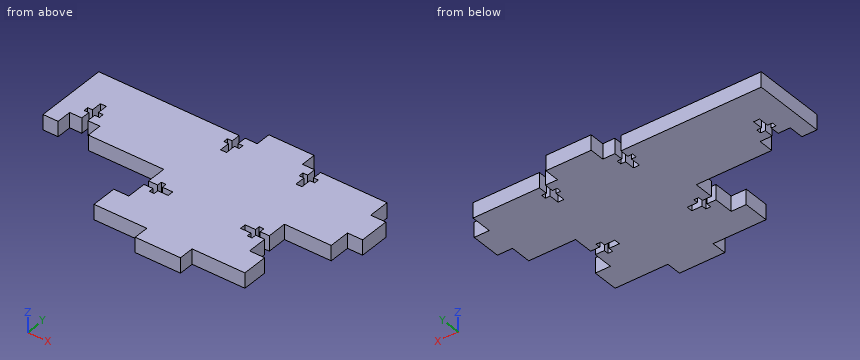
from build123d import *

# Parameters (mm, degrees)
BOSS_EXTRUDE1_DEPTH = 6.35
SKETCH2_W           = 12.7
SKETCH2_H           = 6.35
CUT_EXTRUDE1_DEPTH  = 7.35
CUT_EXTRUDE2_DEPTH  = 7.35
CUT_EXTRUDE3_DEPTH  = 7.35


with BuildPart() as part:
    # Sketch1 → Boss-Extrude1 (new body)
    with BuildSketch(Plane.XY):
        Polygon((0, -6.35), (19.05, -6.35), (19.05, 0), (34.925, 0), (41.275, 0), (41.275, 10.795), (34.925, 10.795), (34.925, 29.845), (54.61, 29.845), (54.61, 38.735), (60.96, 38.735), (60.96, 51.435), (54.61, 51.435), (54.61, 60.325), (34.925, 60.325), (19.05, 60.325), (19.05, 66.675), (0, 66.675), (0, 60.325), (-15.875, 60.325), (-66.675, 60.325), (-66.675, 29.845), (-15.875, 29.845), (-15.875, 10.795), (-22.225, 10.795), (-22.225, 0), (-15.875, 0), (0, 0), align=None)
    extrude(amount=BOSS_EXTRUDE1_DEPTH)

    # Sketch2 → Cut-Extrude1 (cut, through all)
    with BuildSketch(Plane.XY.offset(6.35)):
        with Locations((-53.975, 33.02)):
            Rectangle(SKETCH2_W, SKETCH2_H)
    extrude(amount=-CUT_EXTRUDE1_DEPTH, mode=Mode.SUBTRACT)

    # Sketch3 → Cut-Extrude2 (cut, through all)
    with BuildSketch(Plane.XY.offset(6.35)):
        Polygon((-15.875, 21.57), (-15.875, 19.07), (-12.065, 19.07), (-12.065, 17.07), (-10.065, 17.07), (-10.065, 19.07), (-5.715, 19.07), (-5.715, 21.57), (-10.065, 21.57), (-10.065, 23.57), (-12.065, 23.57), (-12.065, 21.57), align=None)
        Polygon((34.925, 21.57), (34.925, 19.07), (31.115, 19.07), (31.115, 17.07), (29.115, 17.07), (29.115, 19.07), (24.765, 19.07), (24.765, 21.57), (29.115, 21.57), (29.115, 23.57), (31.115, 23.57), (31.115, 21.57), align=None)
    extrude(amount=-CUT_EXTRUDE2_DEPTH, mode=Mode.SUBTRACT)

    # Sketch5 → Cut-Extrude3 (cut, through all)
    with BuildSketch(Plane.XY.offset(6.35)):
        Polygon((-3.1, 56.515), (-3.1, 54.515), (-5.1, 54.515), (-5.1, 50.165), (-7.6, 50.165), (-7.6, 54.515), (-9.6, 54.515), (-9.6, 56.515), (-7.6, 56.515), (-7.6, 60.325), (-5.1, 60.325), (-5.1, 56.515), align=None)
        Polygon((26.65, 60.325), (26.65, 56.515), (28.65, 56.515), (28.65, 54.515), (26.65, 54.515), (26.65, 50.165), (24.15, 50.165), (24.15, 54.515), (22.15, 54.515), (22.15, 56.515), (24.15, 56.515), (24.15, 60.325), align=None)
        Polygon((-52.725, 42.005), (-50.725, 42.005), (-50.725, 40.005), (-52.725, 40.005), (-52.725, 36.195), (-55.225, 36.195), (-55.225, 40.005), (-57.225, 40.005), (-57.225, 42.005), (-55.225, 42.005), (-55.225, 46.355), (-52.725, 46.355), align=None)
    extrude(amount=-CUT_EXTRUDE3_DEPTH, mode=Mode.SUBTRACT)


solid = part.part
The listing builds one solid part. Answer for the finished solid, in the listing's coordinates (mm). Round coordinates to 2 decimals unless told otherwise and drop trailing zeros. Loops run counter-clockwise (first coordinate to the right, second up) from the corner with the lowest first, then second, coordinate; pieces in that order, holes last. Notation, with made-up numbers: M 14.25,14 L 69.25,14 A10 ccw 69.25,30 Z; hole C 36.5,-27.75 d9. An arc over 180 degrees is marked long. Return JSON: item names as keys, results as strings.
Q1. Find section A-A, the plane y = 32.5. Determine the outline of the cut face in (x, z) (3 decimals), plus the area to 3 significant figures.
Results list:
{"outline": "M -66.675,0 L -60.325,0 L -60.325,6.35 L -66.675,6.35 Z; M -47.625,0 L 54.61,0 L 54.61,6.35 L -47.625,6.35 Z", "area": "690 mm2"}
Q2. Each of these flat-tipped pins is pushed along its axis until it touches: pin 1 Ø1 at (y, z) = (12, 1.5) entering from +X (3 decimals); pin 2 Ø3.5 at (x, z) = (26.5, 2) entering from -Y; pin 3 Ø0.6 at (y, z) = (18, 4.5) entering from -X (3 decimals). Where does it stop, or does it pass through?
Results list:
{"pin 1": "stops at x = 34.925", "pin 2": "stops at y = 0", "pin 3": "stops at x = -15.875"}
Q3. Find the intervals of material crossed by line 1 along X through (y, z) = (18, 5) (3 decimals); line 2 along Y through (x, z) = (-13, 5) (3 decimals); line 3 along X through (y, z) = (58.5, 2.5) (3 decimals), in increasing order. Write a range as from..to.
Results list:
{"line 1": "x = -15.875..-12.065, -10.065..29.115, 31.115..34.925", "line 2": "y = 0..19.07, 21.57..60.325", "line 3": "x = -66.675..-7.6, -5.1..24.15, 26.65..54.61"}
Q4. Find section B-B, the plane x = 32.5. Determine the outline of the cut face in (y, z) (3 decimals), plus the area to 3 significant figures.
Results list:
{"outline": "M 0,0 L 19.07,0 L 19.07,6.35 L 0,6.35 Z; M 21.57,0 L 60.325,0 L 60.325,6.35 L 21.57,6.35 Z", "area": "367 mm2"}
